Design review of the part built by this model. Coordinates are the model's own, in mm. A direction names the side the tool comes from. Coordinates: 2 decimals unless noted, no trailing zeros. Loops run counter-clockwise (first coordinate to the right, second up) from the corner with the lowest first, then second, coordinate; pieces in that order, holes last. Notation, with made-up numbers: (49.5, -33) -> (58.5, -33) arc R18 ccw to (58.5, -29) -> close; hole circle Ø2 at (49, -3). An arc over 180 degrees is marked (long way). Use CSV: the item, a comma, the result in double quotes.
```python
from build123d import *

# Parameters (mm, degrees)
SKETCH1_W           = 34.925
SKETCH1_H           = 12.7
BOSS_EXTRUDE1_DEPTH = 2.54
FILLET1_R           = 0.635
SHELL1_START        = 0.635
SHELL1_OUTLINE_W    = 1.905
SHELL1_OUTLINE_H    = 11.43
SHELL1_DEPTH        = 33.655
SKETCH2_R           = 2.54
BOSS_EXTRUDE2_DEPTH = 1.905


# Read off the part's stored shape, not the designer's step: Shell1
with BuildPart() as part:
    # Sketch1 → Boss-Extrude1 (new body)
    with BuildSketch(Plane(origin=(0, 0, 0), x_dir=(1, 0, 0), z_dir=(0, 1, 0))):
        with Locations((17.4625, 6.35)):
            Rectangle(SKETCH1_W, SKETCH1_H)
    extrude(amount=BOSS_EXTRUDE1_DEPTH)

    # Fillet1
    fillet1_edges = [part.edges().sort_by_distance(p)[0] for p in [
        (0, 1.27, -12.7),
        (34.925, 1.27, -12.7),
        (34.925, 1.27, 0),
        (0, 1.27, 0),
    ]]
    fillet(fillet1_edges, radius=FILLET1_R)

    # Shell1 outline → Shell1 (cut)
    with BuildSketch(Plane.YZ.offset(SHELL1_START)):
        with Locations((0.9525, -6.35)):
            Rectangle(SHELL1_OUTLINE_W, SHELL1_OUTLINE_H)
    extrude(amount=SHELL1_DEPTH, mode=Mode.SUBTRACT)

    # Sketch2 → Boss-Extrude2 (add)
    with BuildSketch(Plane(origin=(0, 1.905, 0), x_dir=(-1, 0, 0), z_dir=(0, -1, 0))):
        with Locations(Location((-17.4625, 6.35, 0), (0, 0, 270))):
            Circle(SKETCH2_R)
    extrude(amount=BOSS_EXTRUDE2_DEPTH)


solid = part.part
```
Item 1: Machinability: for faces 4 (the face through (17.351, 0.966, -8.888)), 5 (the face through (17, 1, 0)), which of the approach directions +Z, -Z, +X, -X, +Y, -Y give a long, thin tool a straight path to every point of the face, cutting with its end or side? Answer none if there is none.
Checked values:
face 4,"-Y"
face 5,"+Z, +X, -X, +Y, -Y"
Item 2: Clearance check with a flat-ended pin moving along its axis: pin 1 (2 mm diameter, centred on x = 26, z = -4.5, fed in from -Y) (3 decimals). State where the tip first meets the part, or that it passes through.
Checked values:
pin 1,"y = 1.905"
Item 3: Add section C-C (x = 13). Give the boundary of the cut face in (y, z) (3 decimals).
Checked values:
outline,"(0, -12.7) -> (2.54, -12.7) -> (2.54, 0) -> (0, 0) -> (0, -0.635) -> (1.905, -0.635) -> (1.905, -12.065) -> (0, -12.065) -> close"
Item 4: Add section B-B (z = -6.35). Give the boundary of the cut face in (x, y) (1 decimal), then the cut area to 3 significant figures.
Checked values:
outline,"(0, 0) -> (0.6, 0) -> (0.6, 1.9) -> (14.9, 1.9) -> (14.9, 0) -> (20, 0) -> (20, 1.9) -> (34.3, 1.9) -> (34.3, 0) -> (34.9, 0) -> (34.9, 2.5) -> (0, 2.5) -> close"
area,"34.3 mm^2"
Item 5: Add section D-D (x = 16.5). Give the boundary of the cut face in (y, z) (3 decimals).
Checked values:
outline,"(0, -12.7) -> (2.54, -12.7) -> (2.54, 0) -> (0, 0) -> (0, -0.635) -> (1.905, -0.635) -> (1.905, -3.999) -> (0, -3.999) -> (0, -8.701) -> (1.905, -8.701) -> (1.905, -12.065) -> (0, -12.065) -> close"
Item 6: Draft analysis for pull direction X (two halves, no side actions). For faces 1 (the face through (17, 1.905, -9)), 2 (the face through (0, 1, -6)), 3 (the face through (12.2, 0, -0.3)), state which applies: pulls with the +X half, pulls with the -X half, needs draft (parallel to the pull), parting line crosses it, or undercut.
Checked values:
face 1,"undercut"
face 2,"pulls with the -X half"
face 3,"needs draft"
Item 7: To check wall thickness, follow line 1 along Z through (x, y) = (18.5, 1.2) (3 decimals); line 2 along Z through (x, y) = (32, 1.55) (3 decimals); line 3 along X through (y, z) = (0.45, -10.25) (3 decimals). State the ranges of each line that lie inside material, in increasing order.
Checked values:
line 1,"-12.7 to -12.065, -8.668 to -4.032, -0.635 to 0"
line 2,"-12.7 to -12.065, -0.635 to 0"
line 3,"0 to 0.635, 34.29 to 34.925"
Item 8: Add section A-A (y = 0.75). State how many separate pieces and enclosed holes the cut face has, then the cut area to 3 significant figures.
Checked values:
separate pieces,"2"
enclosed holes,"1"
area,"78.8 mm^2"
